Answer from the drawing. Dimensions are ordinates in mm from the lowest x, y and z of the part. A direction names the side the tool comes from. Coordinates: 2 decimals unless noted, no trailing zeros. Write each loop counter-clockwise with the first axis right and the second up, starting at its lowest first coordinate (ties: lowest second). Pieces come first, ordered by that corner, then holes. Notation, with made-up numbers: (5.5, -33.5) - (21.5, -33.5) arc R18 ccw to (21.5, -17.5) - close; hole circle Ø7 at (80, -23.75). An arc over 180 degrees is marked (long way). Answer as a JSON object with one key per item and string values. Group by question number.
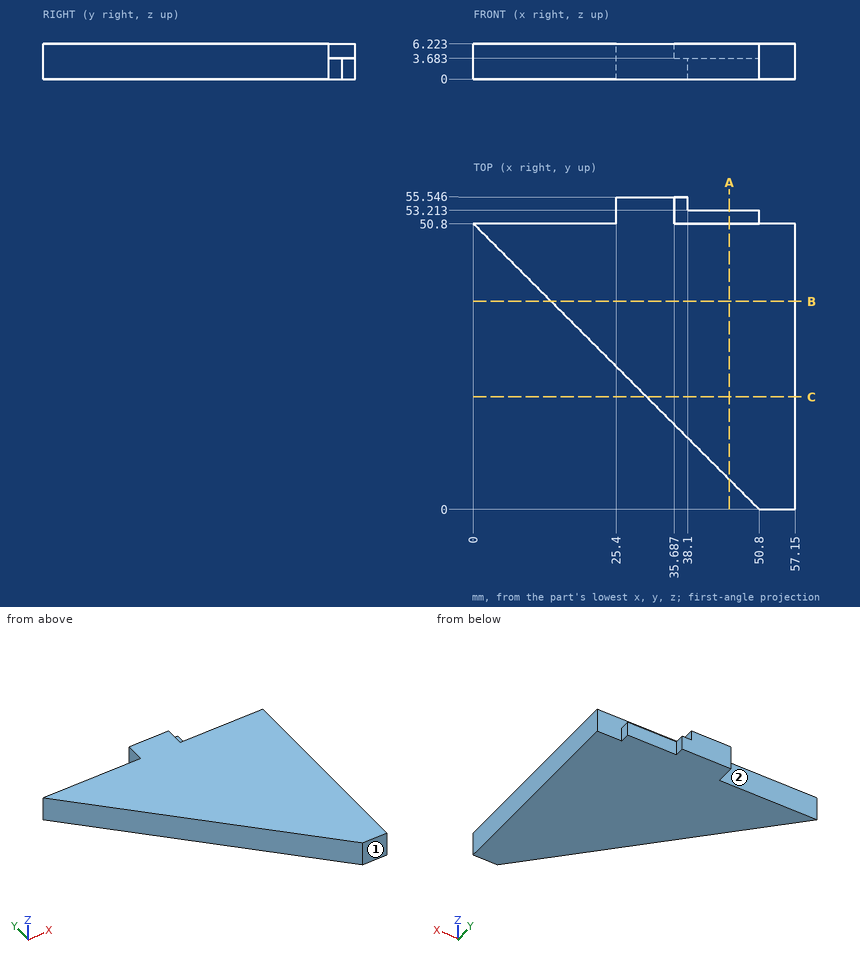
Q1. A tool of negligible diameter and unlimited length cuts with its end or side. For the marked faces 1 and 2, from which of +Z, -Z, +X, -X, +Y, -Y can it reach the whole face along a straight path? Write none if from no direction.
Q2. Section A-A on x = 45.5 is taken. Determine the outline of the cut face in (y, z).
Q3. Section B-B on y = 37 is taken. Determine the outline of the cut face in (x, z), plus the area to 3 significant figures.
Q4. Consider L1, parallel to Y at x = 53, z = 4; L2, parallel to X at y = 36, z = 4.25; L3, parallel to X at y = 49.5, z = 5.75. Determine where each line is inside the solid, lowest interval first. Write a range as from..to.
Q5. Section C-C on y = 20 is taken. Determine the outline of the cut face in (x, z).
Q6. Flat-ended cylindrical pins translate along their axes: pin 1 Ø1.9 at (x, z) = (49.5, 2) entering from +Y; pin 2 Ø2 at (y, z) = (47.5, 1) entering from -X; pin 3 Ø1.3 at (y, z) = (53.5, 5.5) entering from +X. Find the tip coordinate at first contact, or state that the pin passes through.
Numbers:
{
 "1": {"face 1": "+Z, -Z, +X, -X, -Y", "face 2": "+Z, -Z, -X, +Y"},
 "2": {"outline": "(5.3, 0) - (53.21, 0) - (53.21, 3.68) - (50.8, 3.68) - (50.8, 6.22) - (5.3, 6.22) - close"},
 "3": {"outline": "(13.8, 0) - (57.15, 0) - (57.15, 6.22) - (13.8, 6.22) - close", "area": "270 mm²"},
 "4": {"L1": "y = 0..50.8", "L2": "x = 14.8..57.15", "L3": "x = 1.3..57.15"},
 "5": {"outline": "(30.8, 0) - (57.15, 0) - (57.15, 6.22) - (30.8, 6.22) - close"},
 "6": {"pin 1": "stops at y = 53.21", "pin 2": "stops at x = 2.3", "pin 3": "stops at x = 35.69"}
}
